Here's the drawing with two shaded views (mm, measured from the low corner). I have some questions. A direction names the side the tool comes from. Coordinates: 2 decimals unless noted, no trailing zeros. Write each loop counter-clockwise with the first axis right and the second up, starting at its lowest first coordinate (ties: lowest second). Pieces come first, ordered by that corner, then holes.
Item 1: I want a section at A-A on x = 19.05. Please give me the cut outline in (y, z) (3 decimals).
Item 2: I want a section at B-B on z = 3.81. Please give me the cut outline in (x, y) (3 decimals).
Item 3: I want a section at C-C on y = 2.5. Please give me the cut outline in (x, z) (3 decimals), then the cut area to 3 significant figures.
Item 4: For P1, Ø2, axis at y = 9.5, z = 27, coming from the +X side; P2, Ø19, axis at x = 16, z = 22.5, coming from the -Y side, each with a flat end and sliding along its axis, tell me the tip position at first contact or that it passes through.
Item 5: Which directions (+Z, -Z, +X, -X, +Y, -Y) give clear straight access to the entire face, cutting with the end or side of a thin tool? Please do the marked faces 1 and 2.
Item 6: Thinking about a two-plate mould opening in X: for the marked faces 3, 4, 5 and 6, which applies, +X half, -X half, draft (parallel to the pull), parting line (faces both ways), or undercut?
Item 7: I want a section at D-D on y = 7.25. Please give me the cut outline in (x, z).
Item 8: If I drill on probe 1 along X at (y, z) = (16.25, 33.5); probe 2 along Y at (x, z) = (27, 12); probe 3 along X at (y, z) = (5.75, 5), over which ranges is the centre line in solid material (lowest first)?
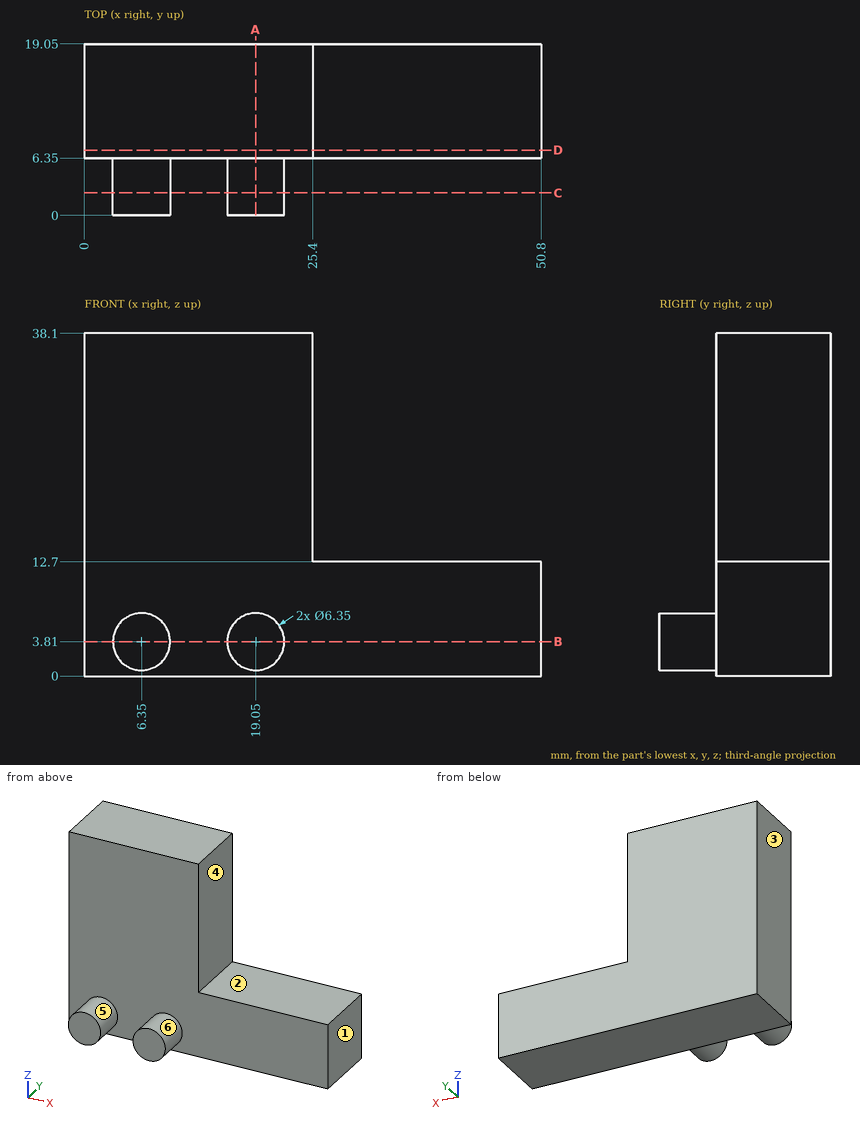
Response values:
1. outline: (0, 0.635) - (6.35, 0.635) - (6.35, 0) - (19.05, 0) - (19.05, 38.1) - (6.35, 38.1) - (6.35, 6.985) - (0, 6.985) - close
2. outline: (0, 6.35) - (3.175, 6.35) - (3.175, 0) - (9.525, 0) - (9.525, 6.35) - (15.875, 6.35) - (15.875, 0) - (22.225, 0) - (22.225, 6.35) - (50.8, 6.35) - (50.8, 19.05) - (0, 19.05) - close
3. outline: circle Ø6.35 at (6.35, 3.81); circle Ø6.35 at (19.05, 3.81)
3. area: 63.3 mm2
4. P1: stops at x = 25.4
4. P2: stops at y = 6.35
5. face 1: +Z, -Z, +X, +Y, -Y
5. face 2: +Z, +X, +Y, -Y
6. face 3: -X half
6. face 4: +X half
6. face 5: undercut
6. face 6: undercut
7. outline: (0, 0) - (50.8, 0) - (50.8, 12.7) - (25.4, 12.7) - (25.4, 38.1) - (0, 38.1) - close
8. probe 1: x = 0 to 25.4
8. probe 2: y = 6.35 to 19.05
8. probe 3: x = 3.41 to 9.29, 16.11 to 21.99
